Here's how the part is built. I have some questions about the finished solid (model axes, mm). A direction names the side the tool comes from. Coordinates: 2 decimals unless noted, no trailing zeros. Write each loop counter-clockwise with the first axis right and the second up, starting at its lowest first coordinate (ties: lowest second). Pieces come first, ordered by that corner, then holes.
Item 1: For faces 4 (the face through (2, 22.225, 2)), 5 (the face through (-0.54, 23.83, -73.77)), which set-ups out of +Z, -Z, +X, -X, +Y, -Y let a thin tool reach every point of the face, with its end or its side?
Item 2: I'm going to push flat-ended pins straight in: pin 1 Ø2 at (x, y) = (8, 0) entering from -Z; pin 2 Ø8 at (x, z) = (0, -50.8) entering from +Y. Where does each tip first touch, or does it pass through?
Item 3: If we section it at A-A (y = 0): Please give me the cut outline in (x, z) (3 decimals).
Item 4: If I drill on line 1 (Y direction, x = 0.25, z = -82) (3 decimals); line 2 (X direction, y = 10, z = 13.5) (3 decimals); line 3 (Y direction, x = 11.2, z = -101.6), over which ranges is the centre line in solid material (lowest first)?
Item 5: We'd pull the mould along Z, two halves only. Please class faces 1 (the face through (-10, -2, 114.3)), 2 (the face through (11.09, -0.95, -103.9)), 3 (the face through (-12.7, 0, 2)): +Z half, -Z half, draft (parallel to the pull), parting line (faces both ways), or undercut.
Item 6: If we section it at C-C (x = -6.75): Please give me the cut outline in (y, z) (3 decimals), then the cut area to 3 significant figures.
Item 7: If we section it at B-B (z = 76.2): Please give me the cut outline in (x, y) (3 decimals).
from build123d import *

# Parameters (mm, degrees)
SKETCH1_W           = 25.4
SKETCH1_H           = 50.8
SKETCH1_W_2         = 19.05
SKETCH1_H_2         = 44.45
BOSS_EXTRUDE1_DEPTH = 114.3
SKETCH2_R           = 2.4892
CUT_EXTRUDE1_DEPTH  = 51.8
SKETCH3_R           = 2.4892
CUT_EXTRUDE2_DEPTH  = 26.4


with BuildPart() as part:
    # Sketch1 → Boss-Extrude1 (new body, symmetric)
    with BuildSketch(Plane.XY):
        Rectangle(SKETCH1_W, SKETCH1_H)
        Rectangle(SKETCH1_W_2, SKETCH1_H_2, mode=Mode.SUBTRACT)
    extrude(amount=BOSS_EXTRUDE1_DEPTH, both=True)

    # Sketch2 → Cut-Extrude1 (cut, through all)
    with BuildSketch(Plane(origin=(0, 25.4, 0), x_dir=(1, 0, 0), z_dir=(0, 1, 0))):
        with Locations((0, -101.6)):
            Circle(SKETCH2_R)
        with Locations((0, -76.2)):
            Circle(SKETCH2_R)
        with Locations((0, -50.8)):
            Circle(SKETCH2_R)
        with Locations((0, -25.4)):
            Circle(SKETCH2_R)
        Circle(SKETCH2_R)
        with Locations((0, 25.4)):
            Circle(SKETCH2_R)
        with Locations((0, 50.8)):
            Circle(SKETCH2_R)
        with Locations((0, 76.2)):
            Circle(SKETCH2_R)
        with Locations((0, 101.6)):
            Circle(SKETCH2_R)
    extrude(amount=-CUT_EXTRUDE1_DEPTH, mode=Mode.SUBTRACT)

    # Sketch3 → Cut-Extrude2 (cut, through all)
    with BuildSketch(Plane.ZY.offset(12.7)):
        with Locations((101.6, 0)):
            Circle(SKETCH3_R)
        with Locations((101.6, -12.7)):
            Circle(SKETCH3_R)
        with Locations((101.6, 12.7)):
            Circle(SKETCH3_R)
    cut_extrude2 = extrude(amount=-CUT_EXTRUDE2_DEPTH, mode=Mode.SUBTRACT)

    # Mirror1: Cut-Extrude2 across plane
    add(cut_extrude2.mirror(Plane.XY), mode=Mode.SUBTRACT)


solid = part.part
Answer list:
1. face 4: +Z, -Z
1. face 5: +Y, -Y
2. pin 1: passes through
2. pin 2: stops at y = 25.4
3. outline: (-12.7, -114.3) - (-9.525, -114.3) - (-9.525, -104.089) - (-12.7, -104.089) - close; (-12.7, -99.111) - (-9.525, -99.111) - (-9.525, 99.111) - (-12.7, 99.111) - close; (-12.7, 104.089) - (-9.525, 104.089) - (-9.525, 114.3) - (-12.7, 114.3) - close; (9.525, -114.3) - (12.7, -114.3) - (12.7, -104.089) - (9.525, -104.089) - close; (9.525, -99.111) - (12.7, -99.111) - (12.7, 99.111) - (9.525, 99.111) - close; (9.525, 104.089) - (12.7, 104.089) - (12.7, 114.3) - (9.525, 114.3) - close
4. line 1: y = -25.4 to -22.225, 22.225 to 25.4
4. line 2: x = -12.7 to -9.525, 9.525 to 12.7
4. line 3: y = -25.4 to -15.19, -10.21 to -2.49, 2.49 to 10.21, 15.19 to 25.4
5. face 1: +Z half
5. face 2: undercut
5. face 3: draft
6. outline: (-25.4, -114.3) - (-22.225, -114.3) - (-22.225, 114.3) - (-25.4, 114.3) - close; (22.225, -114.3) - (25.4, -114.3) - (25.4, 114.3) - (22.225, 114.3) - close
6. area: 1,450 mm2
7. outline: (-12.7, -25.4) - (-2.489, -25.4) - (-2.489, -22.225) - (-9.525, -22.225) - (-9.525, 22.225) - (-2.489, 22.225) - (-2.489, 25.4) - (-12.7, 25.4) - close; (2.489, -25.4) - (12.7, -25.4) - (12.7, 25.4) - (2.489, 25.4) - (2.489, 22.225) - (9.525, 22.225) - (9.525, -22.225) - (2.489, -22.225) - close
